Could you check a few things on this model? Use its own coordinates, in mm. Round coordinates to 2 decimals unless told otherwise and drop trailing zeros. Write each loop counter-clockwise with the first axis right and the second up, starting at its lowest first coordinate (ties: lowest second). Pieces come first, ordered by that corner, then holes. Notation, with made-up numbers: (64, 22.25) -> (117, 22.25) arc R16 cw to (117, 37.25) -> close; hole circle Ø5 at (61, 54.5). An arc over 180 degrees is marked (long way). Answer in a Markdown table with one row per item.
from build123d import *

# Parameters (mm, degrees)
SKETCH_1_R      = 1.6
EXTRUDE_1_DEPTH = 2


with BuildPart() as part:
    # Эскиз1 → Бобышка-Вытянуть1 (new body)
    with BuildSketch(Plane.XY):
        with BuildLine():
            Line((0, -4.241468847), (2.758531153, -7))
            Line((2.758531153, -7), (15.329410732, -19.570879578))
            Line((15.329410732, -19.570879578), (15.429120422, -19.670589268))
            ThreePointArc((15.429120422, -19.670589268), (19.670589268, -19.570879578), (19.570879578, -15.329410732))
            Line((19.570879578, -15.329410732), (13, -8.758531153))
            Line((13, -8.758531153), (13, 6))
            Line((13, 6), (-1.758531153, 6))
            Line((-1.758531153, 6), (-15.329410732, 19.570879578))
            Line((-15.329410732, 19.570879578), (-15.429120422, 19.670589268))
            ThreePointArc((-15.429120422, 19.670589268), (-19.670589268, 19.570879578), (-19.570879578, 15.329410732))
            Line((-19.570879578, 15.329410732), (0, -4.241468847))
        make_face()
        with Locations((17.5, -17.5)):
            Circle(SKETCH_1_R, mode=Mode.SUBTRACT)
        with Locations((-17.5, 17.5)):
            Circle(SKETCH_1_R, mode=Mode.SUBTRACT)
    extrude(amount=EXTRUDE_1_DEPTH)


solid = part.part
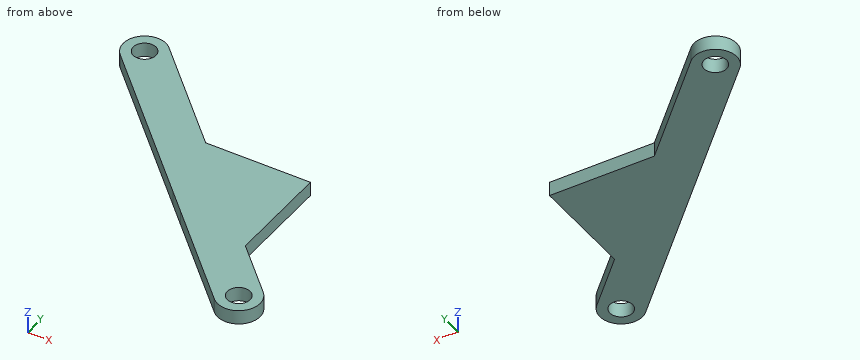
1) Imagine slicing it at A-A, the plane z = 1.3. Please give me the cut outline in (x, y).
Findings:
| item | result |
|---|---|
| outline | (-19.57, 15.33) -> (15.43, -19.67) arc R3 ccw to (19.57, -15.33) -> (13, -8.76) -> (13, 6) -> (-1.76, 6) -> (-15.43, 19.67) arc R3 ccw to start; hole circle Ø3.2 at (-17.5, 17.5); hole circle Ø3.2 at (17.5, -17.5) |
2) Imagine slicing it at D-D, the plane x = 8. Please give me the cut outline in (y, z).
Findings:
| item | result |
|---|---|
| outline | (-12.24, 0) -> (6, 0) -> (6, 2) -> (-12.24, 2) -> close |
3) For pin 1 (3.5 mm diameter, centred on x = 17.5, y = -17.5, fed in from -Z); pin 2 (0.6 mm diameter, centred on y = -4, z = 0.5, fed in from +X); pin 3 (1 mm diameter, centred on x = -9.5, z = 1.5, fed in from -Y), each with a flat end and sliding along its axis, tell me the tip position at first contact or that it passes through.
Findings:
| item | result |
|---|---|
| pin 1 | stops at z = 0 |
| pin 2 | stops at x = 13 |
| pin 3 | stops at y = 4.76 |
4) Please list where these lines run through material, in increasing order: line 1 (Y direction, x = 17.5, z = 1); line 2 (Y direction, x = -17.5, z = 0.9); line 3 (X direction, y = 12, z = 0.55).
Findings:
| item | result |
|---|---|
| line 1 | y = -20.5 to -19.1, -15.9 to -13.26 |
| line 2 | y = 13.26 to 15.9, 19.1 to 20.5 |
| line 3 | x = -16.24 to -7.76 |
5) Imagine slicing it at B-B, the plane y = -17.5. Please give me the cut outline in (x, z), plus the area to 3 significant figures.
Findings:
| item | result |
|---|---|
| outline | (13.26, 0) -> (15.9, 0) -> (15.9, 2) -> (13.26, 2) -> close; (19.1, 0) -> (20.5, 0) -> (20.5, 2) -> (19.1, 2) -> close |
| area | 8.08 mm^2 |
